Geometry check sheet. Reference: drawing and pictorial views, mm from the part's lowest x, y, z. A direction names the side the tool comes from. Give positions to 0.01 mm unless a question says otherwise; leave off trailing zeros. Order: outer loops, then holes, each group sorted by start corner. A loop starts at its lowest first (then second) coordinate and runs counter-clockwise, first axis right, second up. Notation, with made-up numbers: M 3.5,17 L 57.5,17 A33 cw 57.5,53 Z; hole C -18.75,56.5 d1. An arc over 180 degrees is marked long. Answer as CSV lines item,"result".
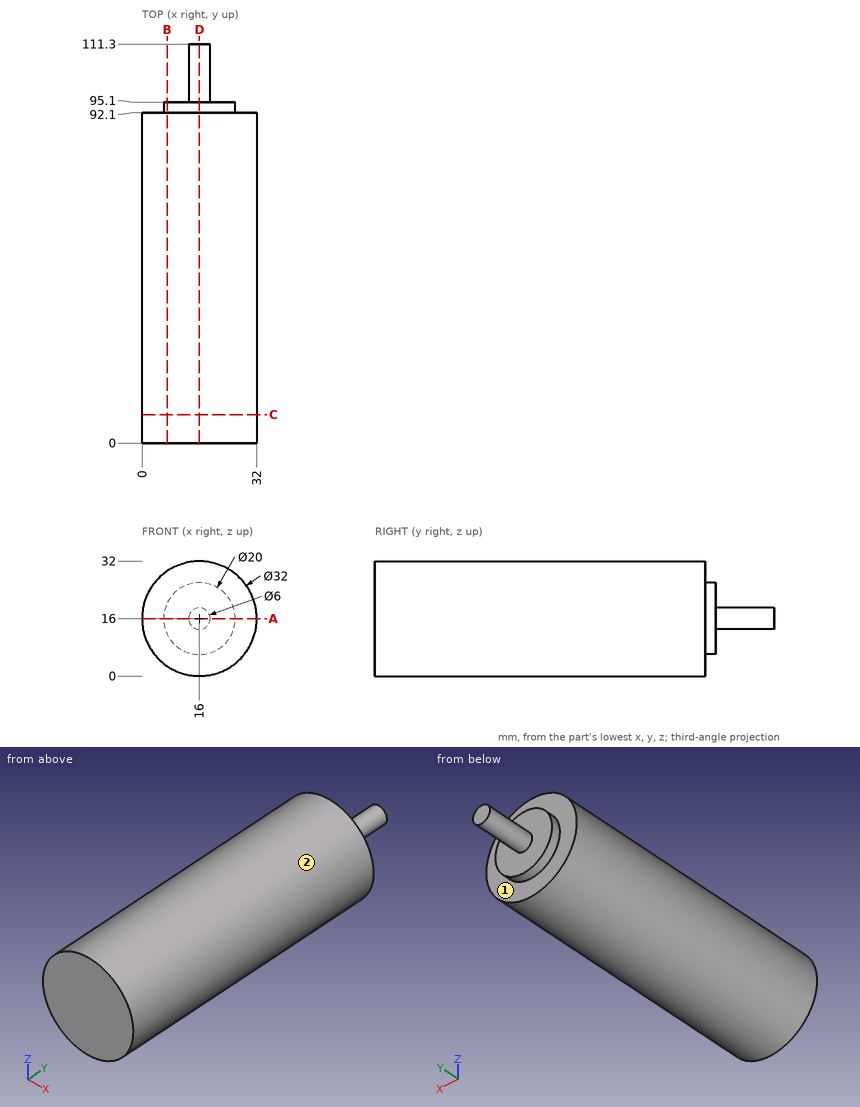
(1) Section check D-D on x = 16. Enter the section's corners in (y, z), then the cut area to 3 significant figures.
The answers:
outline,"M 0,0 L 92.1,0 L 92.1,6 L 95.1,6 L 95.1,13 L 111.3,13 L 111.3,19 L 95.1,19 L 95.1,26 L 92.1,26 L 92.1,32 L 0,32 Z"
area,"3,100 mm2"
(2) Section check B-B on x = 7. Enter the section's corners in (y, z).
The answers:
outline,"M 0,2.77 L 92.1,2.77 L 92.1,11.64 L 95.1,11.64 L 95.1,20.36 L 92.1,20.36 L 92.1,29.23 L 0,29.23 Z"
(3) Section check A-A on z = 16. Enter the section's corners in (x, y).
The answers:
outline,"M 0,0 L 32,0 L 32,92.1 L 26,92.1 L 26,95.1 L 19,95.1 L 19,111.3 L 13,111.3 L 13,95.1 L 6,95.1 L 6,92.1 L 0,92.1 Z"
(4) Section check C-C on y = 8. Enter the section's corners in (x, z).
The answers:
outline,"C 16,16 d32"
(5) Material ranges on line 1 (Y direction, x = 11, z = 4.5); line 2 (Y direction, x = 9, z = 12); line 3 (Z direction, x = 15, y = 46.5), recorded low to high.
The answers:
line 1,"y = 0 to 92.1"
line 2,"y = 0 to 95.1"
line 3,"z = 0.03 to 31.97"
(6) Tool access check on the marked faces 1 and 2. Record the directions out of +Z, -Z, +X, -X, +Y, -Y that give a thin tool (end or side, any length) a straight path to the whole face; none if there is none.
The answers:
face 1,"+Y"
face 2,"+Y, -Y"
(7) Gauge pin test, flat ends, axial feed: P1, Ø5, axis at x = 12, z = 25.5, coming from the +Y side; P2, Ø2, axis at x = 23.5, y = 72.5, coming from the +Z side; P3, Ø6, axis at x = 12.5, z = 11.5, coming from the +Y side; P4, Ø4, axis at x = 6.5, y = 85.5, coming from the -Z side. Record the tip position at first contact, or that the pin passes through.
The answers:
P1,"stops at y = 95.1"
P2,"stops at z = 30.62"
P3,"stops at y = 111.3"
P4,"stops at z = 1.87"
